```python
from build123d import *

# Parameters (mm, degrees)
F0_R            = 40
F1_DEPTH        = 10
F2_R            = 4.8873689042
F3_DEPTH        = 25
F3_COPIES_COUNT = 5
F4_R            = 10
F5_DEPTH        = 25


# Not quite as in the source:
# - a pattern or mirror of a feature is missing from the dataset's text; its kind, count and spacing are read off the source's solid


with BuildPart() as f1:
    # F0 (on Front) → F1 (new body)
    with BuildSketch(Plane.XZ):
        Circle(F0_R)
    extrude(amount=F1_DEPTH)

    # F2 (on face) → F3 (cut)
    with BuildSketch(Plane.XZ.offset(10)):
        with Locations((0, 27.5)):
            Circle(F2_R)
    f3 = extrude(amount=-F3_DEPTH, mode=Mode.SUBTRACT)

    # F3_copies: F3 ×5 about axis
    f3_copies_axis = Axis((0, 0, 0), (0, 1, 0))
    for i in range(1, F3_COPIES_COUNT):
        add(f3.rotate(f3_copies_axis, i * 360 / F3_COPIES_COUNT), mode=Mode.SUBTRACT)

    # F4 (on face) → F5 (cut)
    with BuildSketch(Plane.XZ.offset(10)):
        Circle(F4_R)
    extrude(amount=-F5_DEPTH, mode=Mode.SUBTRACT)


solid = f1.part
```
The listing builds one solid part. Answer for the finished solid, in the listing's coordinates (mm). Coordinates: 2 decimals unless noted, no trailing zeros. Loops run counter-clockwise (first coordinate to the right, second up) from the corner with the lowest first, then second, coordinate; pieces in that order, holes last. Notation, with made-up numbers: (8, 30) - (46, 30) arc R17 ccw to (46, 53) - close; hole circle Ø10 at (-1.75, 43.25). An arc over 180 degrees is marked (long way). Use a Markdown table: item, result. Add a question column.
1) The part is cut by section D-D, the plane z = 7. Give the vertices of the cut face in (x, y), and give its area (3 significant figures).
2) The part is cut by section B-B, the plane z = -3.5. Give the vertices of the cut face in (x, y).
3) Find the intervals of material crossed by line 1 (Z direction, x = 3, y = -3.25); line 2 (Z direction, x = 3.5, y = -6.25); line 3 (X direction, y = -1, z = 8), in increasing order.
4) Given pin 1 (5 mm diameter, centred on y = -5, z = 12, fed in from +X); pin 2 (8 mm diameter, centred on x = -10.5, z = -26.5, fed in from +Y); pin 3 (8 mm diameter, centred on x = -26.15, z = 8.5, fed in from +Y); pin 4 (3 mm diameter, centred on y = -5.5, z = -27.5, fed in from +X), each flat-ended and moving along its own axis, determine where each tip first touches the part or whether it passes through.
5) The part is cut by section A-A, the plane x = 0. Give the vertices of the cut face in (y, z), and give its area (3 significant figures).
6) The part is cut by section C-C, the plane y = -3. Give the vertices of the cut face in (x, z), and give its area (3 significant figures).
7) The mould has two halves that part along X. Classify faces 1 (the cylindrical face through (-8.67, -4.93, -39.05)), 2 (the cylindrical face through (-30.409, -5.07, 6.093)), 3 (the flat face through (8, 0, -8)): released by +X, released by -X, zero draft, split by the parting line, or undercut.
Here are the results:
| question | item | result |
|---|---|---|
| 1 | outline | (-39.38, -10) - (-30.81, -10) - (-30.81, 0) - (-39.38, 0) - close; (-21.5, -10) - (-7.14, -10) - (-7.14, 0) - (-21.5, 0) - close; (7.14, -10) - (21.5, -10) - (21.5, 0) - (7.14, 0) - close; (30.81, -10) - (39.38, -10) - (39.38, 0) - (30.81, 0) - close |
| 1 | area | 459 mm^2 |
| 2 | outline | (-39.85, -10) - (-9.37, -10) - (-9.37, 0) - (-39.85, 0) - close; (9.37, -10) - (39.85, -10) - (39.85, 0) - (9.37, 0) - close |
| 3 | line 1 | z = -39.89 to -9.54, 9.54 to 23.64, 31.36 to 39.89 |
| 3 | line 2 | z = -39.85 to -9.37, 9.37 to 24.09, 30.91 to 39.85 |
| 3 | line 3 | x = -39.19 to -31.02, -21.29 to -6, 6 to 21.29, 31.02 to 39.19 |
| 4 | pin 1 | stops at x = 38.86 |
| 4 | pin 2 | stops at y = 0 |
| 4 | pin 3 | passes through |
| 4 | pin 4 | stops at x = 30.4 |
| 5 | outline | (-10, -40) - (0, -40) - (0, -10) - (-10, -10) - close; (-10, 10) - (0, 10) - (0, 22.61) - (-10, 22.61) - close; (-10, 32.39) - (0, 32.39) - (0, 40) - (-10, 40) - close |
| 5 | area | 502 mm^2 |
| 6 | outline | circle Ø80 at (0, 0); hole circle Ø9.77 at (-26.15, 8.5); hole circle Ø9.77 at (-16.16, -22.25); hole circle Ø20 at (0, 0); hole circle Ø9.77 at (0, 27.5); hole circle Ø9.77 at (16.16, -22.25); hole circle Ø9.77 at (26.15, 8.5) |
| 6 | area | 4,340 mm^2 |
| 7 | face 1 | split by the parting line |
| 7 | face 2 | undercut |
| 7 | face 3 | zero draft |
